Can you work these out from the model? Positions are in its coordinate system, mm. A direction names the side the tool comes from. Coordinates: 2 decimals unless noted, no trailing zeros. Order: outer loops, then holes, each group sorted by start corner. A loop starts at its lowest first (then second) coordinate and runs counter-clockwise, first axis right, second up. Notation, with made-up numbers: (-7.75, 67.25) -> (3.25, 67.25) arc R20 ccw to (3.25, 88.25) -> close; hole circle Ø8 at (44.5, 80). An arc over 180 degrees is marked (long way). Answer in a Markdown table with one row per item. Add a question column.
1. Imagine slicing it at C-C on x = 54. Write out the boundary of the cut face in (y, z).
2. Will this pin go through, and if not, where does the flat tip stop? pin 1 (2 mm diameter, centred on x = 19, z = 4, fed in from -Y).
3. On a 3-axis mill with a long thin cutter (end or side, diameter ignored), from which of +Z, -Z, +X, -X, +Y, -Y can I reach the whole of each face in a straight line? I mean faces 1 (the face through (60, -4, 4)), 2 (the face through (-9.63, -1.08, 4.88)), 3 (the face through (-20, 0, 0)). Say none if no direction works.
4. If I drill on line 1 along Z through (x, y) = (65, -3); line 2 along Z through (x, y) = (-8, 0.25); line 3 along X through (y, z) = (-3.25, 4), over which ranges is the centre line in solid material (lowest first)? Write a range as [from, to].
5. Imagine slicing it at A-A on z = 0. Write out the boundary of the cut face in (x, y).
Autodesk Inventor part; units mm, degrees
ref_plane "YZ Plane" through (0, 0, 0) normal (1, 0, 0) x (0, 1, 0)
ref_plane "XY Plane" through (0, 0, 0) normal (0, 0, 1) x (1, 0, 0)
sketch "Sketch1" plane through (0, 0, 0) normal (0, 0, 1) x (1, 0, 0)
  line L0 (0, 0) -> (60, 0)
  line L1 (60, 0) -> (60, 6)
  line L2 (60, 6) -> (0, 6)
  line L3 (0, 6) -> (0, 0)
  line L4 (0, 0) -> (0, 5)
  line L5 (0, 5) -> (-20, 5)
  line L6 (-20, 5) -> (-20, 0)
  line L7 (-20, 0) -> (0, 0)
  line L8 (60, 5) -> (80, 5)
  line L9 (80, 5) -> (80, 0)
  line L10 (80, 0) -> (60, 0)
  dimension "d0" = 60
  dimension "d1" = 6
  dimension "d3" = 5
  dimension "d4" = 20
  dimension "d5" = 20
revolve "Revolution1" add sketch "Sketch1" angle 360 about axis through (0, 0, 0) along (1, 0, 0)
thread "Thread1"
chamfer "Chamfer1" distance 1 angle 45 2 edges at (-20, -5, 0) (80, -5, 0)
ref_plane "Work Plane1" through (30, 0, 0) normal (1, 0, 0) x (0, 0, -1)
properties part number "Large Gear Shaft"
Answers follow:
| question | item | result |
|---|---|---|
| 1 | outline | circle Ø12 at (0, 0) |
| 2 | pin 1 | stops at y = -5.2 |
| 3 | face 1 | +X |
| 3 | face 2 | -X |
| 3 | face 3 | +Z, -Z, -X, +Y, -Y |
| 4 | line 1 | z = [-4, 4] |
| 4 | line 2 | z = [-4.99, 4.99] |
| 4 | line 3 | x = [0, 60] |
| 5 | outline | (-20, -4) -> (-19, -5) -> (0, -5) -> (0, -6) -> (60, -6) -> (60, -5) -> (79, -5) -> (80, -4) -> (80, 4) -> (79, 5) -> (60, 5) -> (60, 6) -> (0, 6) -> (0, 5) -> (-19, 5) -> (-20, 4) -> close |
